Geometry check sheet. Reference: the model listing, model coordinates, mm. Face numbers are marked on the shaded views. A direction names the side the tool comes from. Coordinates: 2 decimals unless noted, no trailing zeros. Write each loop counter-clockwise with the first axis right and the second up, starting at its lowest first coordinate (ties: lowest second). Pieces come first, ordered by that corner, then holes.
from build123d import *

# Parameters (mm, degrees)
SKETCH_W            = 24.202
SKETCH_H            = 41.474
PAD_DEPTH           = 9.33
CHAMFER_SIZE        = 0.7
POCKET_DEPTH        = 4.33
SKETCH002_R         = 0.955
POCKET001_DEPTH     = 6.771
POCKET002_DEPTH     = 8.734
SKETCH007_W         = 1.36
SKETCH007_H         = 2.46
SKETCH007_H_2       = 1.96
POCKET005_DEPTH     = 0.5
SKETCH004_W         = 9.11
SKETCH004_H         = 5
PAD001_DEPTH        = 4.08
SKETCH005_W         = 12.16
SKETCH005_H         = 3.66
POCKET003_DEPTH     = 8.839
SKETCH006_W         = 12.16
SKETCH006_H         = 4.82
POCKET004_DEPTH     = 8.839
SKETCH008_W         = 1.96
SKETCH008_H         = 3.36
SKETCH008_W_2       = 1.76
SKETCH008_H_2       = 1.76
POCKET006_DEPTH     = 2.06
POCKET007_DEPTH     = 5.771
SKETCH010_R         = 1.23
POCKET008_DEPTH     = 8.831
LINEARPATTERN_COUNT = 9
LINEARPATTERN_PITCH = 2.54
SKETCH011_W         = 7.98
SKETCH011_H         = 2.96
POCKET009_DEPTH     = 6.467


with BuildPart() as part:
    # Sketch → Pad (new body)
    with BuildSketch(Plane.XY.offset(-2.56)):
        with Locations((9.271, 19.431)):
            Rectangle(SKETCH_W, SKETCH_H)
    extrude(amount=PAD_DEPTH)

    # Chamfer
    chamfer_edges = [part.edges().sort_by_distance(p)[0] for p in [
        (-2.83, -1.306, 2.105),
        (21.372, -1.306, 2.105),
        (9.271, -1.306, -2.56),
        (9.271, -1.306, 6.77),
        (21.372, 40.168, 2.105),
        (21.372, 19.431, -2.56),
        (21.372, 19.431, 6.77),
        (-2.83, 40.168, 2.105),
        (9.271, 40.168, -2.56),
        (9.271, 40.168, 6.77),
        (-2.83, 19.431, -2.56),
        (-2.83, 19.431, 6.77),
    ]]
    chamfer(chamfer_edges, length=CHAMFER_SIZE)

    # Sketch001 → Pocket (cut)
    with BuildSketch(Plane.XY.offset(-0.06)):
        with BuildLine():
            Line((-0.33, 2.21), (0.686, 1.194))
            Line((0.686, 1.194), (17.856, 1.194))
            Line((17.856, 1.194), (18.872, 2.21))
            Line((18.872, 2.21), (18.872, 36.652))
            Line((18.872, 36.652), (17.856, 37.668))
            Line((17.856, 37.668), (0.686, 37.668))
            Line((0.686, 37.668), (-0.33, 36.652))
            Line((-0.33, 36.652), (-0.33, 22.784))
            Line((-0.33, 22.784), (1.27, 22.784))
            ThreePointArc((1.7, 22.354), (1.574056, 22.658056), (1.27, 22.784))
            Line((1.7, 22.354), (1.7, 18.54))
            ThreePointArc((1.27, 18.11), (1.574056, 18.235944), (1.7, 18.54))
            Line((1.27, 18.11), (-0.33, 18.11))
            Line((-0.33, 18.11), (-0.33, 2.21))
        make_face()
    extrude(amount=POCKET_DEPTH, mode=Mode.SUBTRACT)

    # Sketch002 → Pocket001 (cut, through all)
    with BuildSketch(Plane.XY):
        with Locations((15.24, 5.08)):
            Circle(SKETCH002_R)
    extrude(amount=POCKET001_DEPTH, mode=Mode.SUBTRACT)

    # Sketch003 → Pocket002 (cut, through all)
    with BuildSketch(Plane.XZ.offset(-7.427)):
        with BuildLine():
            Line((5.194, 4.27), (11.824, 4.27))
            ThreePointArc((13.064, 3.03), (12.700812, 3.906812), (11.824, 4.27))
            Line((13.064, 3.03), (13.064, 2.23))
            ThreePointArc((11.824, 0.99), (12.700812, 1.353188), (13.064, 2.23))
            Line((11.824, 0.99), (5.194, 0.99))
            ThreePointArc((3.954, 2.23), (4.317188, 1.353188), (5.194, 0.99))
            Line((3.954, 2.23), (3.954, 3.03))
            ThreePointArc((5.194, 4.27), (4.317188, 3.906812), (3.954, 3.03))
        make_face()
    extrude(amount=POCKET002_DEPTH, mode=Mode.SUBTRACT)

    # Sketch007 → Pocket005 (cut)
    with BuildSketch(Plane.XY):
        with Locations((4.189, 6.907)):
            Rectangle(SKETCH007_W, SKETCH007_H)
        with Locations((4.189, 2.727)):
            Rectangle(SKETCH007_W, SKETCH007_H_2)
        with Locations((12.829, 2.727)):
            Rectangle(SKETCH007_W, SKETCH007_H_2)
        with Locations((12.829, 6.907)):
            Rectangle(SKETCH007_W, SKETCH007_H)
    extrude(amount=-POCKET005_DEPTH, mode=Mode.SUBTRACT)

    # Sketch004 → Pad001 (join)
    with BuildSketch(Plane.XY.offset(2.69)):
        with Locations((8.509, 10.007)):
            Rectangle(SKETCH004_W, SKETCH004_H)
    extrude(amount=PAD001_DEPTH)

    # Sketch005 → Pocket003 (cut, through all)
    with BuildSketch(Plane.XZ.offset(-31.33)):
        with Locations((8.453, 2.83)):
            Rectangle(SKETCH005_W, SKETCH005_H)
    extrude(amount=-POCKET003_DEPTH, mode=Mode.SUBTRACT)

    # Sketch006 → Pocket004 (cut, through all)
    with BuildSketch(Plane.XZ.offset(-31.33)):
        with Locations((8.453, 2.25)):
            Rectangle(SKETCH006_W, SKETCH006_H)
    extrude(amount=-POCKET004_DEPTH, mode=Mode.SUBTRACT)

    # Sketch008 → Pocket006 (cut)
    with BuildSketch(Plane.XY):
        with Locations((2.603, 34.427)):
            Rectangle(SKETCH008_W, SKETCH008_H)
        with Locations((14.303, 34.427)):
            Rectangle(SKETCH008_W, SKETCH008_H)
        with Locations((4.953, 32.627)):
            Rectangle(SKETCH008_W_2, SKETCH008_H_2)
        with Locations((7.453, 32.627)):
            Rectangle(SKETCH008_W_2, SKETCH008_H_2)
        with Locations((9.453, 32.627)):
            Rectangle(SKETCH008_W_2, SKETCH008_H_2)
        with Locations((11.953, 32.627)):
            Rectangle(SKETCH008_W_2, SKETCH008_H_2)
    extrude(amount=-POCKET006_DEPTH, mode=Mode.SUBTRACT)

    # Sketch009 → Pocket007 (cut, through all)
    with BuildSketch(Plane.XY.offset(1)):
        Polygon((13.433, 33.125), (19.333, 33.125), (19.333, 6.575), (16.383, 6.575), (13.433, 6.575), align=None)
    extrude(amount=POCKET007_DEPTH, mode=Mode.SUBTRACT)

    # Sketch010 → Pocket008 (cut, through all)
    with BuildSketch(Plane.XY.offset(-2.06)):
        with Locations((16.383, 9.525)):
            Circle(SKETCH010_R)
    pocket008 = extrude(amount=POCKET008_DEPTH, mode=Mode.SUBTRACT)

    # LinearPattern: Pocket008 ×9
    with Locations(*[(0, i * LINEARPATTERN_PITCH, 0) for i in range(1, LINEARPATTERN_COUNT)]):
        add(pocket008, mode=Mode.SUBTRACT)

    # Sketch011 → Pocket009 (cut, through all)
    with BuildSketch(Plane.YZ.offset(3.636)):
        with Locations((13.462, -0.3)):
            Rectangle(SKETCH011_W, SKETCH011_H)
    extrude(amount=-POCKET009_DEPTH, mode=Mode.SUBTRACT)


solid = part.part
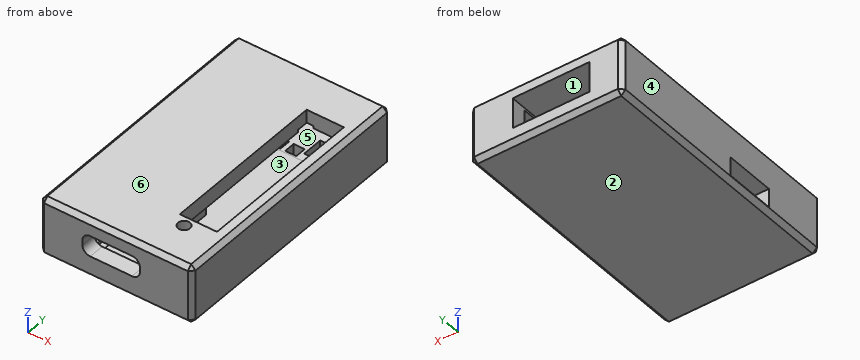
1. Draft check along X on the marked faces 1, 2, 3 and 4. Enter one of: released by +X, released by -X, zero draft, split by the parting line, or undercut.
Computed values:
face 1: undercut
face 2: zero draft
face 3: undercut
face 4: released by -X
2. Gauge pin test, flat end, axial feed: pin 1 Ø3 at (x, y) = (16.383, 24.765) entering from +Z. Record the tip position at first contact, or that the pin passes through.
Computed values:
pin 1: stops at z = -0.06
3. Thickness scan on line 1 along Z through (x, y) = (10.25, 14); line 2 along Y through (x, z) = (15.24, 5.75) (3 decimals); line 3 along Y through (x, z) = (17, 4.5) (3 decimals). Record the ranges inside material, lowest first.
Computed values:
line 1: z = -2.56 to -0.06, 4.27 to 6.77
line 2: y = -1.306 to 4.125, 6.035 to 6.575, 33.125 to 40.168
line 3: y = -1.306 to 6.575, 33.125 to 40.168
4. Sectioned sample at A-A, the plane y = 5.08. Record the boundary of the cut face in (x, z) (3 decimals).
Computed values:
outline: (-2.83, -1.86) - (-2.13, -2.56) - (20.672, -2.56) - (21.372, -1.86) - (21.372, 6.07) - (20.672, 6.77) - (16.195, 6.77) - (16.195, 4.27) - (18.872, 4.27) - (18.872, -0.06) - (-0.33, -0.06) - (-0.33, 4.27) - (14.285, 4.27) - (14.285, 6.77) - (-2.13, 6.77) - (-2.83, 6.07) - close
5. Access from +Z, -Z, +X, -X, +Y, -Y to the whole of each face (thin tool, end or side, straight path). Record for the marked faces 5 and 6.
Computed values:
face 5: +Y
face 6: +Z, +X, -X, +Y, -Y
